Here's how the part is built. I have some questions about the finished solid (model axes, mm). Round coordinates to 2 decimals unless told otherwise and drop trailing zeros. Order: outer loops, then holes, each group sorted by start corner. A loop starts at its lowest first (then second) coordinate and runs counter-clockwise, first axis right, second up. Notation, with made-up numbers: M 7.5,72.25 L 28.5,72.25 A22 cw 28.5,94.25 Z; hole C 81.5,28 d7. An arc over 180 degrees is marked long. Answer as CSV lines item,"result". Start each with the question number.
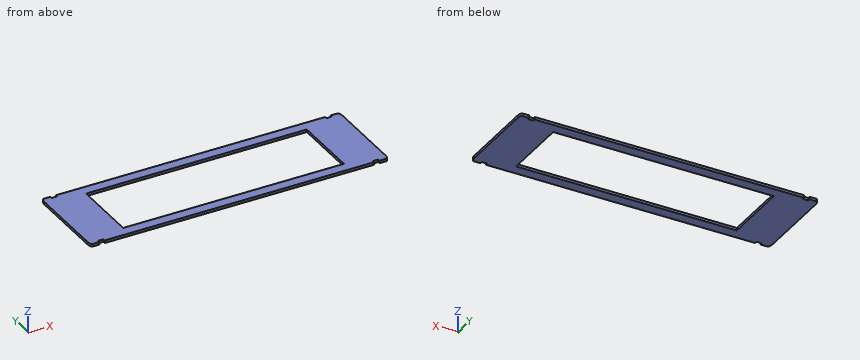
```python
from build123d import *

# Parameters (mm, degrees)
SKETCH_1_W               = 270
SKETCH_1_H               = 79
EXTRUDE_1_DEPTH          = 2.4
SKETCH_2_W               = 200
SKETCH_2_H               = 60
CUT_EXTRUDE_1_DEPTH      = 141.680524594
FILLET_1_SIZE            = 5
FILLET_1_SIZE_2          = 1.8
SKETCH_3_W               = 5
SKETCH_3_H               = 2
CUT_EXTRUDE_2_DEPTH      = 141.68052472
MIRROR_2_COPY_1_SKETCH_W = 5
MIRROR_2_COPY_1_SKETCH_H = 2
MIRROR_2_COPY_1_DEPTH    = 141.68052472


with BuildPart() as part:
    # 草图1 → 凸台-拉伸1 (new body)
    with BuildSketch(Plane.XY):
        Rectangle(SKETCH_1_W, SKETCH_1_H)
    extrude(amount=EXTRUDE_1_DEPTH)

    # 草图2 → 切除-拉伸1 (cut, through all)
    with BuildSketch(Plane.XY.offset(2.4)):
        Rectangle(SKETCH_2_W, SKETCH_2_H)
    extrude(amount=-CUT_EXTRUDE_1_DEPTH, mode=Mode.SUBTRACT)

    # 圆角1
    # an asymmetric fillet: 5, 1.8 mm, written as the material it takes off along each edge
    with BuildSketch(Plane(origin=(135, -39.5, -12.5), x_dir=(0, 1, 0), z_dir=(0, 0, 1))) as fillet_1_piece_1:
        with BuildLine():
            Bezier((FILLET_1_SIZE, 0), (0, 0), (0, FILLET_1_SIZE_2), weights=[1, 0.707106781, 1])
            Line((0, FILLET_1_SIZE_2), (0, 0))
            Line((0, 0), (FILLET_1_SIZE, 0))
        make_face()
    extrude(amount=27.4, mode=Mode.SUBTRACT)
    with BuildSketch(Plane(origin=(135, 39.5, -12.5), x_dir=(-1, 0, 0), z_dir=(0, 0, 1))) as fillet_1_piece_2:
        with BuildLine():
            Bezier((FILLET_1_SIZE_2, 0), (0, 0), (0, FILLET_1_SIZE), weights=[1, 0.707106781, 1])
            Line((0, FILLET_1_SIZE), (0, 0))
            Line((0, 0), (FILLET_1_SIZE_2, 0))
        make_face()
    extrude(amount=27.4, mode=Mode.SUBTRACT)
    with BuildSketch(Plane(origin=(-135, -39.5, -12.5), x_dir=(0, 1, 0), z_dir=(0, 0, 1))) as fillet_1_piece_3:
        with BuildLine():
            Bezier((FILLET_1_SIZE, 0), (0, 0), (0, -FILLET_1_SIZE_2), weights=[1, 0.707106781, 1])
            Line((0, -FILLET_1_SIZE_2), (0, 0))
            Line((0, 0), (FILLET_1_SIZE, 0))
        make_face()
    extrude(amount=27.4, mode=Mode.SUBTRACT)
    with BuildSketch(Plane(origin=(-135, 39.5, -12.5), x_dir=(1, 0, 0), z_dir=(0, 0, 1))) as fillet_1_piece_4:
        with BuildLine():
            Bezier((FILLET_1_SIZE_2, 0), (0, 0), (0, -FILLET_1_SIZE), weights=[1, 0.707106781, 1])
            Line((0, -FILLET_1_SIZE), (0, 0))
            Line((0, 0), (FILLET_1_SIZE_2, 0))
        make_face()
    extrude(amount=27.4, mode=Mode.SUBTRACT)

    # 草图3 → 切除-拉伸2 (cut, through all)
    with BuildSketch(Plane.XY.offset(2.4)):
        with Locations((-124.5, 38.5)):
            Rectangle(SKETCH_3_W, SKETCH_3_H)
    cut_extrude_2 = extrude(amount=-CUT_EXTRUDE_2_DEPTH, mode=Mode.SUBTRACT)

    # 镜向1: 切除-拉伸2 across plane
    add(cut_extrude_2.mirror(Plane.ZX), mode=Mode.SUBTRACT)

    # 镜向2: 切除-拉伸2 across plane
    add(cut_extrude_2.mirror(Plane(origin=(0, 0, 0), x_dir=(0, 0, 1), z_dir=(1, 0, 0))), mode=Mode.SUBTRACT)

    # 镜向2 copy 1 sketch → 镜向2 copy 1 (cut, through all)
    with BuildSketch(Plane(origin=(0, 0, 2.4), x_dir=(-1, 0, 0), z_dir=(0, 0, 1))):
        with Locations((-124.5, 38.5)):
            Rectangle(MIRROR_2_COPY_1_SKETCH_W, MIRROR_2_COPY_1_SKETCH_H)
    extrude(amount=-MIRROR_2_COPY_1_DEPTH, mode=Mode.SUBTRACT)


solid = part.part
```
Item 1: For P1, Ø1.2, axis at x = -124.5, z = 0.5, coming from the +Y side; P2, Ø0.6, axis at y = -38.5, z = 1, coming from the -X side; P3, Ø1, axis at y = -38.5, z = 1, coming from the +X side, each with a flat end and sliding along its axis, tell me the tip position at first contact or that it passes through.
Item 2: If I drill on line 1 along Y through (x, z) = (91, 0.7); line 2 along X through (y, z) = (9.5, 0.4); line 3 along X through (y, z) = (-35, 0.2), over which ranges is the centre line in solid material (lowest first)?
Item 3: If we section it at B-B on y = 10.5: Please give me the cut outline in (x, z).
Item 4: If we section it at A-A on x = 74.5: Please give me the cut outline in (y, z), and give its area (3 significant figures).
Geometry says:
1,P1,"y = 37.5"
1,P2,"x = -134.41"
1,P3,"x = 134.49"
2,line 1,"-39.5 to -30, 30 to 39.5"
2,line 2,"-135 to -100, 100 to 135"
2,line 3,"-134.99 to 134.99"
3,outline,"M -135,0 L -100,0 L -100,2.4 L -135,2.4 Z; M 100,0 L 135,0 L 135,2.4 L 100,2.4 Z"
4,outline,"M -39.5,0 L -30,0 L -30,2.4 L -39.5,2.4 Z; M 30,0 L 39.5,0 L 39.5,2.4 L 30,2.4 Z"
4,area,"45.6 mm²"
